Verification items for this drawing (mm, ordinates from the low corner). A direction names the side the tool comes from. Round coordinates to 2 decimals unless told otherwise and drop trailing zeros. Order: outer loops, then holes, each group sorted by start corner. A loop starts at its lowest first (then second) coordinate and runs counter-clockwise, first axis right, second up. Notation, with made-up numbers: (-5, 82) - (44, 82) arc R6 cw to (44, 86) - close; hole circle Ø9 at (12, -31.5). An arc over 180 degrees is marked (long way). One line per question, with ' | ' between items. Start each with the question number.
Q1. Sectioned sample at C-C, the plane x = 44. Enter the section's corners in (y, z) (3 decimals).
Q2. Sectioned sample at D-D, the plane z = 6.75. Enter the section's corners in (x, y) (3 decimals), then the cut area to 3 significant figures.
Q3. Tool access check on the marked faces 5 and 6. Record the directions out of +Z, -Z, +X, -X, +Y, -Y that give a thin tool (end or side, any length) a straight path to the whole face; none if there is none.
Q4. Material ranges on line 1 along X through (y, z) = (5.25, 3.25) (3 decimals); line 2 along Y through (x, z) = (44, 4.5) (3 decimals); line 3 along Z through (x, y) = (30, 8) (3 decimals), recorded low to high.
Q5. Mould release check, pull along X, two halves, no side actions. Record for the marked faces 1, 2, 3 and 4: +X half, -X half, draft (parallel to the pull), parting line (faces both ways), or undercut.
Q6. Sectioned sample at B-B, the plane z = 2.25. Enter the section's corners in (x, y) (3 decimals), then the cut area to 3 significant figures.
Q7. Gauge pin test, flat ends, axial feed: P1, Ø1.5, axis at x = 43.5, y = 4, coming from the +Z side (3 decimals); P2, Ø1, axis at x = 35, z = 2, coming from the -Y side (3 decimals); P3, Ø5, axis at y = 5.5, z = 4.5, coming from the -X side; P4, Ø3, axis at x = 30, z = 7.5, coming from the -Y side (3 decimals). Record the tip position at first contact, or that the pin passes through.
Q8. Sectioned sample at A-A, the plane y = 2.5. Enter the section's corners in (x, z) (3 decimals).
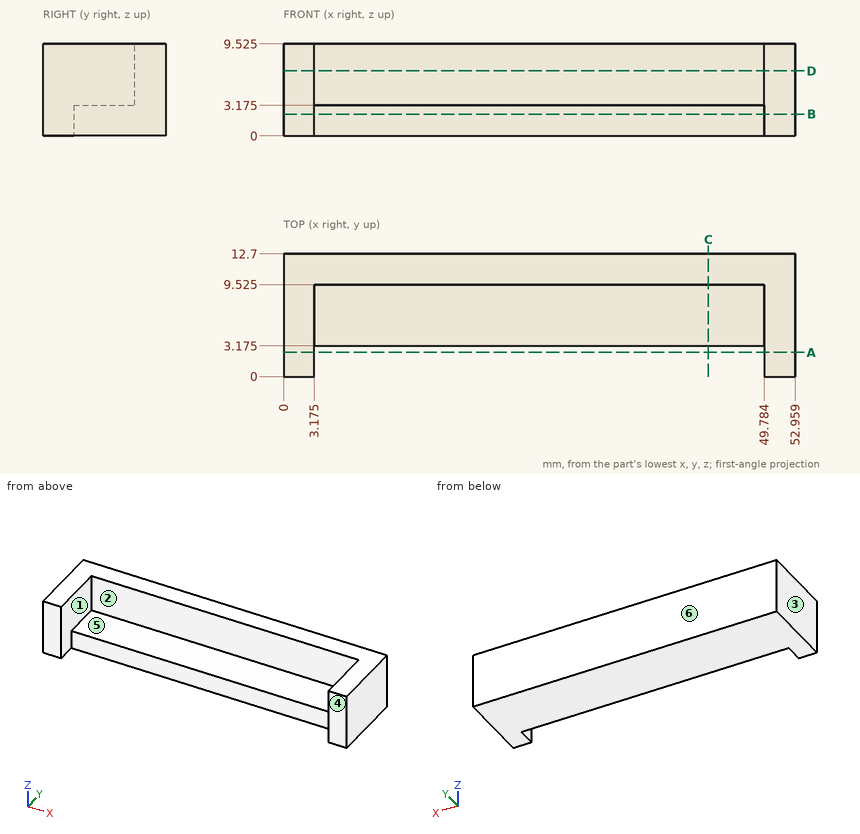
Determined:
1) outline: (3.175, 0) - (12.7, 0) - (12.7, 9.525) - (9.525, 9.525) - (9.525, 3.175) - (3.175, 3.175) - close
2) outline: (0, 0) - (3.175, 0) - (3.175, 9.525) - (49.784, 9.525) - (49.784, 0) - (52.959, 0) - (52.959, 12.7) - (0, 12.7) - close | area: 229 mm2
3) face 5: +Z, -Y | face 6: +Z, -Z, +X, -X, +Y
4) line 1: x = 0 to 3.175, 49.784 to 52.959 | line 2: y = 9.525 to 12.7 | line 3: z = 0 to 3.175
5) face 1: undercut | face 2: undercut | face 3: -X half | face 4: draft
6) outline: (0, 0) - (3.175, 0) - (3.175, 3.175) - (49.784, 3.175) - (49.784, 0) - (52.959, 0) - (52.959, 12.7) - (0, 12.7) - close | area: 525 mm2
7) P1: stops at z = 3.175 | P2: stops at y = 3.175 | P3: stops at x = 0 | P4: stops at y = 9.525
8) outline: (0, 0) - (3.175, 0) - (3.175, 9.525) - (0, 9.525) - close; (49.784, 0) - (52.959, 0) - (52.959, 9.525) - (49.784, 9.525) - close
